from build123d import *

# Parameters (mm, degrees)
F0_W     = 53.975
F0_H     = 1.5875
F1_DEPTH = 280.67
F2_W     = 10.16
F2_H     = 12.7
F2_W_2   = 19.05
F3_DEPTH = 25.4


with BuildPart() as f1:
    # F0 (on Right) → F1 (new body)
    with BuildSketch(Plane.YZ):
        with Locations((-26.9875, 0.79375)):
            Rectangle(F0_W, F0_H)
    extrude(amount=F1_DEPTH)

    # F2 (on face) → F3 (cut)
    with BuildSketch(Plane.XY.offset(1.5875)):
        with Locations((5.08, -6.35)):
            Rectangle(F2_W, F2_H)
        with Locations((271.145, -6.35)):
            Rectangle(F2_W_2, F2_H)
    extrude(amount=-F3_DEPTH, mode=Mode.SUBTRACT)


solid = f1.part
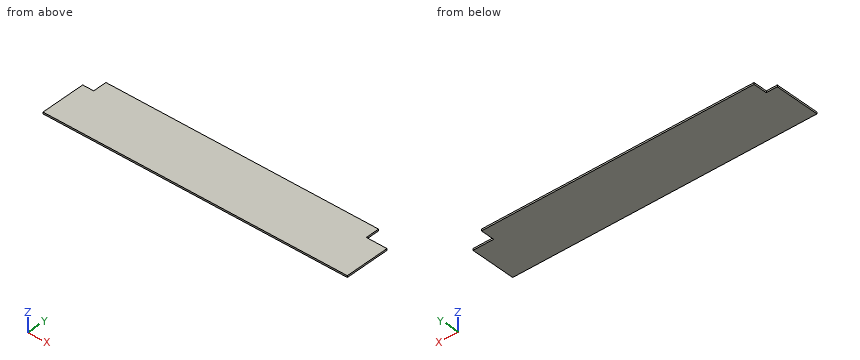
The model under review builds one solid part; all positions refer to its coordinate system, in mm. Round coordinates to 2 decimals unless told otherwise and drop trailing zeros. Loops run counter-clockwise (first coordinate to the right, second up) from the corner with the lowest first, then second, coordinate; pieces in that order, holes last. Notation, with made-up numbers: M 40,26 L 63,26 A15 ccw 63,48 Z; hole C 54.25,79 d10. An arc over 180 degrees is marked long. Answer as a JSON object with one key per item and string values.
Item 1: For line 1 along X through (y, z) = (-5.5, 0.35), list the stretches that pass through material, from the lowest coordinate up.
Check sheet entries:
{"line 1": "10.16 to 261.62"}
Item 2: We need section A-A, the plane z = 0.95. State the section outline as (x, y) points (3 decimals).
Check sheet entries:
{"outline": "M 0,-53.975 L 280.67,-53.975 L 280.67,-12.7 L 261.62,-12.7 L 261.62,0 L 10.16,0 L 10.16,-12.7 L 0,-12.7 Z"}
Item 3: Clearance check with flat-ended pins moving along their axes: P1, Ø0.8, axis at y = -3.5, z = 1, coming from the +X side; P2, Ø0.5, axis at y = -6.5, z = 0.5, coming from the -X side. State where each tip first meets the part, or that it passes through.
Check sheet entries:
{"P1": "x = 261.62", "P2": "x = 10.16"}
Item 4: We need section B-B, the plane y = -7. State the section outline as (x, z) points, and give its area (3 significant figures).
Check sheet entries:
{"outline": "M 10.16,0 L 261.62,0 L 261.62,1.59 L 10.16,1.59 Z", "area": "399 mm2"}
